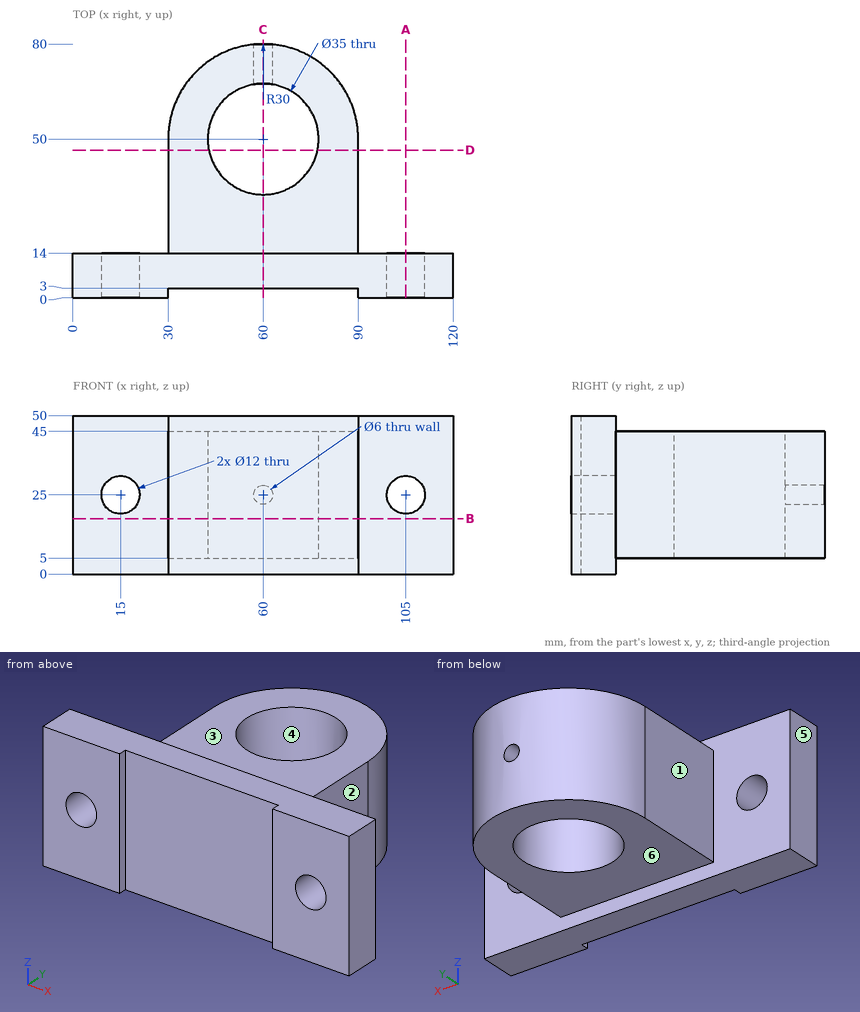
Answer from the drawing. Dimensions are ordinates in mm from the lowest x, y and z of the part. A direction names the side the tool comes from. Give positions to 0.01 mm unless a question says otherwise; leave off trailing zeros. Loops run counter-clockwise (first coordinate to the right, second up) from the corner with the lowest first, then second, coordinate; pieces in that order, holes last. Notation, with made-up numbers: (-8, 87) -> (26, 87) arc R9 ccw to (26, 97) -> close; hole circle Ø3 at (-31, -22.75). An arc over 180 degrees is marked (long way). Use a Markdown table: item, result.
Q1. Section B-B, the plane z = 17.5 is taken. Determine the outline of the cut face in (x, y), then the cut area to 3 significant figures.
Solved:
| item | result |
|---|---|
| outline | (0, 0) -> (30, 0) -> (30, 3) -> (90, 3) -> (90, 0) -> (120, 0) -> (120, 14) -> (90, 14) -> (90, 50) arc R30 ccw to (30, 50) -> (30, 14) -> (0, 14) -> close; hole circle Ø35 at (60, 50) |
| area | 4,110 mm^2 |
Q2. A tool of negligible diameter and unlimited length cuts with its end or side. For the marked faces 1, 2 and 3, from which of +Z, -Z, +X, -X, +Y, -Y can it reach the whole face along a straight path? Write none if from no direction.
Solved:
| item | result |
|---|---|
| face 1 | +Z, -Z, -X, +Y |
| face 2 | +Z, -Z, +X, +Y |
| face 3 | +Z, +X, -X, +Y |
Q3. Find the intervals of material crossed by line 1 along X through (y, z) = (11, 25); line 2 along Z through (x, y) = (84.5, 35.5); line 3 along Y through (x, z) = (22, 40.5), in increasing order.
Solved:
| item | result |
|---|---|
| line 1 | x = 0 to 9, 21 to 99, 111 to 120 |
| line 2 | z = 5 to 45 |
| line 3 | y = 0 to 14 |
Q4. Section C-C, the plane x = 60 is taken. Determine the outline of the cut face in (y, z), then the cut area to 4 significant figures.
Solved:
| item | result |
|---|---|
| outline | (3, 0) -> (14, 0) -> (14, 5) -> (32.5, 5) -> (32.5, 45) -> (14, 45) -> (14, 50) -> (3, 50) -> close; (67.5, 5) -> (80, 5) -> (80, 22) -> (67.5, 22) -> close; (67.5, 28) -> (80, 28) -> (80, 45) -> (67.5, 45) -> close |
| area | 1,715 mm^2 |
Q5. Each of these flat-tipped pins is pushed along its axis until it touches: pin 1 (6 mm diameter, centred on x = 62, y = 30, fed in from +Z); pin 2 (5 mm diameter, centred on x = 67.5, z = 24, fed in from +Y); pin 3 (4 mm diameter, centred on y = 50.5, z = 44, fed in from +X); pin 4 (6 mm diameter, centred on x = 13, z = 30, fed in from -Y). Where does it stop, or does it pass through?
Solved:
| item | result |
|---|---|
| pin 1 | stops at z = 45 |
| pin 2 | stops at y = 79.58 |
| pin 3 | stops at x = 90 |
| pin 4 | stops at y = 0 |
Q6. Section A-A, the plane x = 105 is taken. Determine the outline of the cut face in (y, z), then the cut area to 3 significant figures.
Solved:
| item | result |
|---|---|
| outline | (0, 0) -> (14, 0) -> (14, 19) -> (0, 19) -> close; (0, 31) -> (14, 31) -> (14, 50) -> (0, 50) -> close |
| area | 532 mm^2 |
Q7. Determine the mould class of the marked faces 4, 5 and 6 for opening direction X: pulls with the +X half, pulls with the -X half, needs draft (parallel to the pull), parting line crosses it, or undercut.
Solved:
| item | result |
|---|---|
| face 4 | undercut |
| face 5 | pulls with the -X half |
| face 6 | needs draft |
Q8. Section D-D, the plane y = 46.5 is taken. Determine the outline of the cut face in (x, z), then the cut area to 3 significant figures.
Solved:
| item | result |
|---|---|
| outline | (30, 5) -> (42.85, 5) -> (42.85, 45) -> (30, 45) -> close; (77.15, 5) -> (90, 5) -> (90, 45) -> (77.15, 45) -> close |
| area | 1,030 mm^2 |
